The model under review builds one solid part; all positions refer to its coordinate system, in mm. A direction names the side the tool comes from. Coordinates: 2 decimals unless noted, no trailing zeros. Write each loop counter-clockwise with the first axis right and the second up, starting at its lowest first coordinate (ties: lowest second). Pieces come first, ordered by that corner, then holes. Notation, with made-up numbers: (66, -11) - (122, -11) arc R20 cw to (122, -3) - close; hole circle Ø3 at (-20, 87). An arc over 180 degrees is marked (long way). Return JSON: item names as keys, results as strings. Group by question number.
(1) We need section B-B on x = 8.25. Give the number of separate pieces and of enclosed holes in the cut face, then the cut area to 3 significant figures.
(2) To check wall thickness, follow L1, parallel to Z at x = 9.5, y = 16.75; L2, parallel to Y at x = 3.5, z = 18.5; L3, parallel to Z at x = 4, y = 23.5. State the ranges of each line that lie inside material, in increasing order. Write a range as from..to.
(3) Tool access review of faces 4 (the face through (5.9, 30.002, 47.6)), 5 (the face through (6, 22, -19.747)), 6 (the face through (9, 17.702, 43)): name each direction out of +Z, -Z, +X, -X, +Y, -Y from which nothing blocks a thin tool from reaching the whole face with its end or side.
(4) For pin 1 Ø3 at (x, z) = (4, -24.5) entering from -Y; pin 2 Ø0.6 at (x, z) = (9, 43.5) entering from -Y; pin 3 Ø1.6 at (y, z) = (15, 43) entering from -X; pin 4 Ø0.9 at (x, y) = (9, 15.5) entering from -Z, all flat-tipped, find the tip position at first contact; note any pin that passes through.
(5) We need section D-D on z = 34. State the section outline as (x, y) points.
(6) We need section C-C on z = -19. State the section outline as (x, y) points, then the cut area to 3 significant figures.
(7) Draft analysis for pull direction X (two halves, no side actions). For faces 1 (the face through (10.2, 30.74, 50.74)), 2 (the face through (0.674, 30.742, 55.35)), 3 (the face through (9, 13.602, -17)), state which applies: released by +X, released by -X, zero draft, split by the parting line, or undercut.
(8) We need section A-A on y = 16.75. State the section outline as (x, z) points, then the cut area to 3 significant figures.
```python
from build123d import *

# Parameters (mm, degrees)
BOSS_EXTRUDE1_DEPTH = 12
CUT_EXTRUDE1_DEPTH  = 60.533114979
FILLET1_R           = 5
FILLET2_R           = 2
CHAMFER1_START      = 29
CHAMFER1_DEPTH      = 4
CHAMFER2_SIZE       = 2
SKETCH3_W           = 3
SKETCH3_H           = 4.1
BOSS_EXTRUDE2_DEPTH = 2
SKETCH4_W           = 3
SKETCH4_H           = 4.1
BOSS_EXTRUDE3_DEPTH = 2


with BuildPart() as part:
    # Sketch1 → Boss-Extrude1 (new body)
    with BuildSketch(Plane(origin=(0, 0, 0), x_dir=(0, 0, -1), z_dir=(1, 0, 0))):
        Polygon((-43.352838341, 30.002180144), (17.247161659, 30.002180144), (18.247161659, 29.002180144), (18.247161659, 13.2495019), (19.747161659, 13.2495019), (19.747161659, 30.002180144), (29.747161659, 30.002180144), (29.747161659, 31.502180144), (17.868482003, 31.502180144), (-43.974158684, 31.502180144), (-55.852838341, 31.502180144), (-55.852838341, 30.002180144), (-45.852838341, 30.002180144), (-45.852838341, 13.2495019), (-44.352838341, 13.2495019), (-44.352838341, 29.002180144), align=None)
    extrude(amount=BOSS_EXTRUDE1_DEPTH)

    # Sketch2 → Cut-Extrude1 (cut, through all)
    with BuildSketch(Plane.XZ.offset(-30.002180144)):
        with BuildLine():
            ThreePointArc((4.585460706, 48.752838341), (10.2, 50.852838341), (4.585460706, 52.952838341))
            Line((4.585460706, 52.952838341), (0, 52.952838341))
            Line((0, 52.952838341), (0, 48.752838341))
            Line((0, 48.752838341), (4.585460706, 48.752838341))
        make_face()
        with BuildLine():
            ThreePointArc((4.585460706, -22.647161659), (10.2, -24.747161659), (4.585460706, -26.847161659))
            Line((4.585460706, -26.847161659), (0, -26.847161659))
            Line((0, -26.847161659), (0, -22.647161659))
            Line((0, -22.647161659), (4.585460706, -22.647161659))
        make_face()
    extrude(amount=-CUT_EXTRUDE1_DEPTH, mode=Mode.SUBTRACT)

    # Fillet1
    fillet1_edges = [part.edges().sort_by_distance(p)[0] for p in [
        (12, 30.752180144, -29.747161659),
        (12, 30.752180144, 55.852838341),
    ]]
    fillet(fillet1_edges, radius=FILLET1_R)

    # Fillet2
    fillet2_edges = [part.edges().sort_by_distance(p)[0] for p in [
        (0, 30.752180144, 55.852838341),
        (0, 30.752180144, -29.747161659),
    ]]
    fillet(fillet2_edges, radius=FILLET2_R)

    # Chamfer1: read off the stored shape, not the designer's step
    # Chamfer1 outline → Chamfer1 (cut)
    with BuildSketch(Plane(origin=(0, 0, 0), x_dir=(1, 0, 0), z_dir=(0, 1, 0)).offset(CHAMFER1_START)):
        with BuildLine():
            Line((1.005012563, 26.847161659), (0.010025126, 27.947161659))
            ThreePointArc((0.010025126, 27.947161659), (0.002507854, 27.847287209), (0, 27.747161659))
            Line((0, 27.747161659), (0, 26.847161659))
            Line((0, 26.847161659), (1.005012563, 26.847161659))
        make_face()
        Polygon((0, 22.647161659), (0, 21.647161659), (1, 22.647161659), align=None)
        Polygon((1, -48.752838341), (0, -47.752838341), (0, -48.752838341), align=None)
        with BuildLine():
            ThreePointArc((0, -53.852838341), (0.002507854, -53.952963891), (0.010025126, -54.052838341))
            Line((0.010025126, -54.052838341), (1.005012563, -52.952838341))
            Line((1.005012563, -52.952838341), (0, -52.952838341))
            Line((0, -52.952838341), (0, -53.852838341))
        make_face()
    extrude(amount=CHAMFER1_DEPTH, mode=Mode.SUBTRACT)

    # Chamfer2
    chamfer2_edges = [part.edges().sort_by_distance(p)[0] for p in [
        (0, 13.2495019, 45.102838341),
        (12, 13.2495019, -18.997161659),
        (0, 13.2495019, -18.997161659),
        (12, 13.2495019, 45.102838341),
    ]]
    chamfer(chamfer2_edges, length=CHAMFER2_SIZE)

    # Sketch3 → Boss-Extrude2 (add)
    with BuildSketch(Plane(origin=(0, 0, 44.352838341), x_dir=(-1, 0, 0), z_dir=(0, 0, -1))):
        with Locations((-8.580589258, 15.652180144)):
            Rectangle(SKETCH3_W, SKETCH3_H)
    extrude(amount=BOSS_EXTRUDE2_DEPTH)

    # Sketch4 → Boss-Extrude3 (add)
    with BuildSketch(Plane.XY.offset(-18.247161659)):
        with Locations((8.580589258, 15.652180144)):
            Rectangle(SKETCH4_W, SKETCH4_H)
    extrude(amount=BOSS_EXTRUDE3_DEPTH)


solid = part.part
```
Ans:
{
 "1": {"separate pieces": "3", "enclosed holes": "0", "area": "178 mm²"},
 "2": {"L1": "-19.75..-16.25, 42.35..45.85", "L2": "30..31.5", "L3": "-19.75..-18.25, 44.35..45.85"},
 "3": {"face 4": "+Z, +X, -X, -Y", "face 5": "-Z, +X, -X, -Y", "face 6": "+X, -X"},
 "4": {"pin 1": "through", "pin 2": "y = 13.6", "pin 3": "x = 7.08", "pin 4": "z = -19.75"},
 "5": {"outline": "(0, 30) - (12, 30) - (12, 31.5) - (0, 31.5) - close"},
 "6": {"outline": "(0, 15.25) - (2, 13.25) - (10, 13.25) - (12, 15.25) - (12, 31.5) - (0, 31.5) - close", "area": "215 mm²"},
 "7": {"face 1": "undercut", "face 2": "released by -X", "face 3": "zero draft"},
 "8": {"outline": "(0, -19.75) - (12, -19.75) - (12, -18.25) - (10.08, -18.25) - (10.08, -16.25) - (7.08, -16.25) - (7.08, -18.25) - (0, -18.25) - close; (0, 44.35) - (7.08, 44.35) - (7.08, 42.35) - (10.08, 42.35) - (10.08, 44.35) - (12, 44.35) - (12, 45.85) - (0, 45.85) - close", "area": "48.0 mm²"}
}
